Input: part model. Units: mm. Frame: model coordinates. A direction names the side the tool comes from. Round coordinates to 2 decimals unless told otherwise and drop trailing zeros. Order: outer loops, then holes, each group sorted by start corner. A loop starts at its lowest first (then second) coordinate and runs counter-clockwise, first axis right, second up. Notation, with made-up numbers: (84, 53) -> (102, 53) arc R27 cw to (102, 77) -> close; hole circle Ø3 at (-30.5, -9). An arc over 180 degrees is marked (long way). Use a Markdown table: item, result.
from build123d import *

# Parameters (mm, degrees)
F1_R            = 17.5
F2_DEPTH        = 5
F3_W            = 50
F3_H            = 60
F4_DEPTH        = 30
F5_R            = 8
F6_DEPTH        = 115
F7_R            = 2
F8_DEPTH        = 25
F8_COPIES_COUNT = 3


# Not quite as in the source:
# - a pattern or mirror of a feature is missing from the dataset's text; its kind, count and spacing are read off the source's solid


with BuildPart() as f2:
    # F1 (on offset) → F2 (new body)
    with BuildSketch(Plane.YZ.offset(150)):
        Circle(F1_R)
    extrude(amount=-F2_DEPTH)



with BuildPart() as f4:
    # F3 (on Right) → F4 (new body)
    with BuildSketch(Plane.YZ):
        with Locations((0, 4)):
            Rectangle(F3_W, F3_H)
    extrude(amount=F4_DEPTH)


with BuildPart() as f2_1:
    add(f2.part)

    add(f4.part)  # F6 merges F4
    # F5 (on face) → F6 (join, through all)
    with BuildSketch(Plane(origin=(145, 0, 0), x_dir=(0, -1, 0), z_dir=(-1, 0, 0))):
        Circle(F5_R)
    extrude(amount=F6_DEPTH)

    # F7 (on face) → F8 (cut)
    with BuildSketch(Plane.YZ.offset(150)):
        with Locations((-13, 0)):
            Circle(F7_R)
    f8 = extrude(amount=-F8_DEPTH, mode=Mode.SUBTRACT)

    # F8_copies: F8 ×3 about axis
    f8_copies_axis = Axis((0, 0, 0), (1, 0, 0))
    for i in range(1, F8_COPIES_COUNT):
        add(f8.rotate(f8_copies_axis, i * 360 / F8_COPIES_COUNT), mode=Mode.SUBTRACT)

    # F9: F2 across plane


with BuildPart() as f2_2:
    add(f2_1.part)
    add(f2_1.part.mirror(Plane.YZ))

    # F10: F2 across plane


with BuildPart() as f2_3:
    add(f2_2.part)
    add(f2_2.part.mirror(Plane.YZ))

    # F11: F2 across plane


with BuildPart() as f2_4:
    add(f2_3.part)
    add(f2_3.part.mirror(Plane.YZ))


solid = f2_4.part
1) Draft query along X for faces 6 (the face through (145, 4, -8)), 7 (the face through (0, 0, 34)), 8 (the face through (150, 0, 0)). Return one class per face: released by +X, released by -X, zero draft, split by the parting line, or undercut.
Answer key:
| item | result |
|---|---|
| face 6 | undercut |
| face 7 | zero draft |
| face 8 | released by +X |
2) Cut plane A-A on y = 11. Return loops of the section in (x, z).
Answer key:
| item | result |
|---|---|
| outline | (-150, -13.61) -> (-145, -13.61) -> (-145, 13.61) -> (-150, 13.61) -> close; (-30, -26) -> (30, -26) -> (30, 34) -> (-30, 34) -> close; (145, -13.61) -> (150, -13.61) -> (150, 13.61) -> (145, 13.61) -> close |
3) Cut plane C-C on y = 0. Return loops of the section in (x, z).
Answer key:
| item | result |
|---|---|
| outline | (-150, -17.5) -> (-145, -17.5) -> (-145, -8) -> (-30, -8) -> (-30, -26) -> (30, -26) -> (30, -8) -> (145, -8) -> (145, -17.5) -> (150, -17.5) -> (150, 17.5) -> (145, 17.5) -> (145, 8) -> (30, 8) -> (30, 34) -> (-30, 34) -> (-30, 8) -> (-145, 8) -> (-145, 17.5) -> (-150, 17.5) -> close |
4) Cut plane D-D on z = 5. Return loops of the section in (x, y) (1 decimal).
Answer key:
| item | result |
|---|---|
| outline | (-150, -16.8) -> (-145, -16.8) -> (-145, -6.2) -> (-30, -6.2) -> (-30, -25) -> (30, -25) -> (30, -6.2) -> (145, -6.2) -> (145, -16.8) -> (150, -16.8) -> (150, 16.8) -> (145, 16.8) -> (145, 6.2) -> (30, 6.2) -> (30, 25) -> (-30, 25) -> (-30, 6.2) -> (-145, 6.2) -> (-145, 16.8) -> (-150, 16.8) -> close |
5) Cut plane B-B on x = -77.5. Return loops of the section in (y, z).
Answer key:
| item | result |
|---|---|
| outline | circle Ø16 at (0, 0) |
6) Contact query for flat-ended pins moving along their axis: P1, Ø1.5, axis at y = -4.5, z = 25, coming from the +X side; P2, Ø3, axis at y = 6.5, z = -11.26, coming from the -X side. Output: stop coordinate, or through.
Answer key:
| item | result |
|---|---|
| P1 | stops at x = 30 |
| P2 | stops at x = -30 |
7) Ray query, probe 1 along X at (y, z) = (10, 1); probe 2 along Z at (x, y) = (-148.65, 6.5); probe 3 along X at (y, z) = (6.5, 17). Return the intervals inside material, ascending.
Answer key:
| item | result |
|---|---|
| probe 1 | x = -150 to -145, -30 to 30, 145 to 150 |
| probe 2 | z = -16.25 to -13.26, -9.26 to 9.26, 13.26 to 16.25 |
| probe 3 | x = -30 to 30 |
8) Set-up query: faces 1 (the face through (88.3, 1.73, -7.81)), 2 (the face through (0, 0, -26)), 3 (the face through (147.535, -13.887, -10.648)), 4 (the face through (0, -25, 4)), 5 (the face through (-147.535, -13.887, -10.648)). Return all of +Z, -Z, +X, -X, +Y, -Y with unobstructed straight access to the full face (end or side cutting, diameter ignored); none if empty.
Answer key:
| item | result |
|---|---|
| face 1 | none |
| face 2 | -Z, +X, -X, +Y, -Y |
| face 3 | +X |
| face 4 | +Z, -Z, +X, -X, -Y |
| face 5 | -X |
